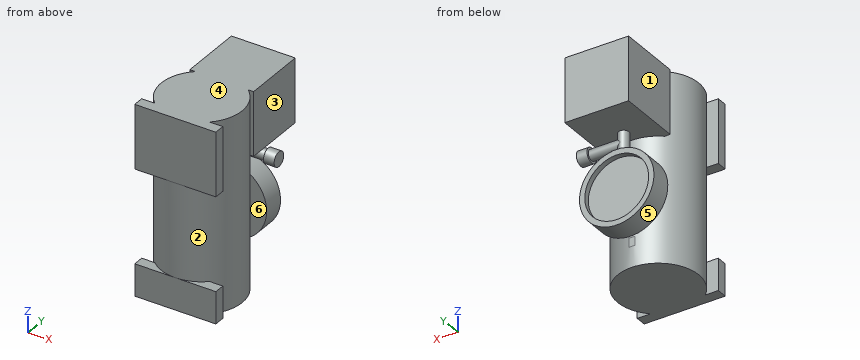
from build123d import *

# Parameters (mm, degrees)
SKETCH1_R           = 38.1
BOSS_EXTRUDE1_DEPTH = 177.8
SKETCH2_W           = 60
SKETCH2_H           = 60
SKETCH2_W_2         = 76.2
SKETCH2_H_2         = 10
BOSS_EXTRUDE2_DEPTH = 60
SKETCH3_R           = 5
BOSS_EXTRUDE3_DEPTH = 20
SKETCH4_W           = 70
SKETCH4_H           = 20
BOSS_EXTRUDE4_DEPTH = 70
CUT_EXTRUDE3_DEPTH  = 22
SKETCH6_R           = 30
CUT_EXTRUDE4_DEPTH  = 5
BOSS_EXTRUDE5_DEPTH = 30
SKETCH8_R           = 5
BOSS_EXTRUDE6_DEPTH = 40
SKETCH9_R           = 6.895484993
BOSS_EXTRUDE7_DEPTH = 10


with BuildPart() as part:
    # Sketch1 → Boss-Extrude1 (new body)
    with BuildSketch(Plane.XY):
        Circle(SKETCH1_R)
    extrude(amount=BOSS_EXTRUDE1_DEPTH)

    # Sketch2 → Boss-Extrude2 (add)
    with BuildSketch(Plane.XY.offset(177.8)):
        with Locations((0, 58.9)):
            Rectangle(SKETCH2_W, SKETCH2_H)
        with Locations((0, -33.1)):
            Rectangle(SKETCH2_W_2, SKETCH2_H_2)
    extrude(amount=-BOSS_EXTRUDE2_DEPTH)

    # Sketch3 → Boss-Extrude3 (add)
    with BuildSketch(Plane(origin=(0, 0, 117.8), x_dir=(-1, 0, 0), z_dir=(0, 0, -1))):
        with Locations((0, 50)):
            Circle(SKETCH3_R)
    extrude(amount=BOSS_EXTRUDE3_DEPTH)

    # Sketch4 → Boss-Extrude4 (add)
    with BuildSketch(Plane(origin=(0, 0, 97.8), x_dir=(-1, 0, 0), z_dir=(0, 0, -1))):
        with Locations((0, 50)):
            Rectangle(SKETCH4_W, SKETCH4_H)
    extrude(amount=BOSS_EXTRUDE4_DEPTH)

    # Sketch5 → Cut-Extrude3 (cut)
    with BuildSketch(Plane(origin=(0, 60, 0), x_dir=(1, 0, 0), z_dir=(0, 1, 0))):
        with BuildLine():
            Line((-5, -106.177349964), (-48.741925114, -106.177349964))
            Line((-48.741925114, -106.177349964), (-48.741925114, -19.422650036))
            Line((-48.741925114, -19.422650036), (48.741925114, -19.422650036))
            Line((48.741925114, -19.422650036), (48.741925114, -106.177349964))
            Line((48.741925114, -106.177349964), (5, -106.177349964))
            Line((5, -106.177349964), (5, -97.441016151))
            ThreePointArc((5, -97.441016151), (0, -27.8), (-5, -97.441016151))
            Line((-5, -97.441016151), (-5, -106.177349964))
        make_face()
    extrude(amount=-CUT_EXTRUDE3_DEPTH, mode=Mode.SUBTRACT)

    # Sketch6 → Cut-Extrude4 (cut)
    with BuildSketch(Plane(origin=(0, 60, 0), x_dir=(1, 0, 0), z_dir=(0, 1, 0))):
        with Locations((0, -62.8)):
            Circle(SKETCH6_R)
    extrude(amount=-CUT_EXTRUDE4_DEPTH, mode=Mode.SUBTRACT)

    # Sketch7 → Boss-Extrude5 (add)
    with BuildSketch(Plane(origin=(0, 0, 0), x_dir=(-1, 0, 0), z_dir=(0, 0, -1))):
        with BuildLine():
            Line((-38.1, -38.1), (0, -38.1))
            ThreePointArc((0, -38.1), (-13.802173742, -35.51211061), (-25.729360661, -28.1))
            Line((-25.729360661, -28.1), (-38.1, -28.1))
            Line((-38.1, -28.1), (-38.1, -38.1))
        make_face()
        with BuildLine():
            Line((38.1, -38.1), (38.1, -28.1))
            Line((38.1, -28.1), (25.729360661, -28.1))
            ThreePointArc((25.729360661, -28.1), (13.802173742, -35.51211061), (0, -38.1))
            Line((0, -38.1), (38.1, -38.1))
        make_face()
    extrude(amount=-BOSS_EXTRUDE5_DEPTH)

    # Sketch8 → Boss-Extrude6 (add)
    with BuildSketch(Plane(origin=(0, 0, 0), x_dir=(0, 0, -1), z_dir=(1, 0, 0))):
        with Locations((-107.620508076, 50)):
            Circle(SKETCH8_R)
    extrude(amount=BOSS_EXTRUDE6_DEPTH)

    # Sketch9 → Boss-Extrude7 (add)
    with BuildSketch(Plane(origin=(40, 0, 0), x_dir=(0, 0, -1), z_dir=(1, 0, 0))):
        with Locations((-107.620508076, 50)):
            Circle(SKETCH9_R)
    extrude(amount=-BOSS_EXTRUDE7_DEPTH)


solid = part.part
Model file for the job. Use its own axes, mm. Face numbers are marked on the shaded views. A direction names the side the tool comes from. Give positions to 0.01 mm unless a question says otherwise; leave off trailing zeros. Order: outer loops, then holes, each group sorted by start corner. A loop starts at its lowest first (then second) coordinate and runs counter-clockwise, first axis right, second up. Notation, with made-up numbers: M 83.25,76 L 103.25,76 A24 cw 103.25,112 Z; hole C -25.75,-29.5 d5. An arc over 180 degrees is marked long. Write item = value, one per line.
Q1. Cut at B-B, the plane z = 17.5. List the corners of the cut face in (x, y).
Derived:
outline = M -38.1,-38.1 L 38.1,-38.1 L 38.1,-28.1 L 25.73,-28.1 A38.1 ccw long -25.73,-28.1 L -38.1,-28.1 Z
Q2. Cut at A-A, the plane z = 62.8. List the corners of the cut face in (x, y).
Derived:
outline = C 0,0 d76.2; M -35,40 L 35,40 L 35,60 L 30,60 L 30,55 L -30,55 L -30,60 L -35,60 Z
Q3. Tool access for the marked faces 1, 2 and 3: list every direction of +Z, -Z, +X, -X, +Y, -Y with a clear straight run to the whole face (end or side of a thin tool).
Derived:
face_1 = +Z, -X, +Y
face_2 = none
face_3 = +Z, +X, +Y
Q4. Flat gauge pins, fed straight in: pin 1 (2 mm diameter, centred on y = 19, z = 142, fed in from +X); pin 2 (3.5 mm diameter, centred on x = 32.5, z = 142.5, fed in from +Y); pin 3 (4 mm diameter, centred on y = 40.5, z = 60, fed in from +X); pin 4 (8 mm diameter, centred on x = -21.5, y = -35, fed in from -Z). Where does each tip first touch, or does it go through?
Derived:
pin_1 = 33.58
pin_2 = 22.5
pin_3 = 34.99
pin_4 = 0
Q5. Two-plate mould, pull along Z, no slides. Class the marked faces 4, 5 and 6: pulls with the +Z half, pulls with the -Z half, needs draft (parallel to the pull), parting line crosses it, or undercut.
Derived:
face_4 = pulls with the +Z half
face_5 = undercut
face_6 = needs draft
Q6. Cut at D-D, the plane y = 32. List the corners of the cut face in (x, z).
Derived:
outline = M -30,117.8 L -20.68,117.8 L -20.68,0 L 20.68,0 L 20.68,117.8 L 30,117.8 L 30,177.8 L -30,177.8 Z
Q7. Cut at C-C, the plane x = 16. List the corners of the cut face in (y, z), then the cut area to 3 significant figures.
Derived:
outline = M -38.1,0 L 34.58,0 L 34.58,117.8 L 88.9,117.8 L 88.9,177.8 L -38.1,177.8 L -38.1,117.8 L -34.58,117.8 L -34.58,30 L -38.1,30 Z; M 40,31.67 L 60,31.67 L 60,37.42 L 55,37.42 L 55,88.18 L 60,88.18 L 60,93.93 L 40,93.93 Z; C 50,107.62 d10
area = 16,900 mm2
Q8. Drill centre lines: line 1 (Z direction, x = 0, y = 58); line 2 (Z direction, x = 27, y = 50); line 3 (X direction, y = 58.1, z = 62.8). Where is each one in solid material? Low to high. Write a range as [from, to].
Derived:
line_1 = [27.8, 32.8], [92.8, 97.8], [117.8, 177.8]
line_2 = [40.53, 85.07], [102.62, 112.62], [117.8, 177.8]
line_3 = [-35, -30], [30, 35]
